The listing builds one solid part. Answer for the finished solid, in the listing's coordinates (mm). Round coordinates to 2 decimals unless told otherwise and drop trailing zeros. Write each loop counter-clockwise with the first axis right and the second up, starting at its lowest first coordinate (ties: lowest second). Pieces come first, ordered by that corner, then holes. Notation, with made-up numbers: (81, 72.5) - (88, 72.5) arc R31 ccw to (88, 101.5) - close; hole circle Ø1 at (30, 70.25). An arc over 180 degrees is marked (long way). Return JSON: item names as keys, results as strings. Group by question number.
(1) Each of these flat-tipped pins is pushed along its axis until it touches: pin 1 (1.5 mm diameter, centred on x = -7.5, y = 1.5, fed in from -Z); pin 2 (1 mm diameter, centred on x = 3.5, y = 0.5, fed in from +Z); pin 3 (1 mm diameter, centred on x = 35, y = 1.5, fed in from -Z). Where does it stop, or does it pass through?
(2) Find the intervals of material crossed by line 1 along Z through (x, y) = (-46.75, 0.7); line 2 along Z through (x, y) = (46.75, 2); line 3 along Z through (x, y) = (-18, 1.4), in increasing order. Write a range as [from, to].
(3) Section D-D, the plane x = -24 is taken. Write down the section's boundary in (y, z), then the cut area to 3 significant figures.
(4) Section B-B, the plane y = 1.6 is taken. Write down the section's boundary in (x, z), then the cut area to 3 significant figures.
(5) Section A-A, the plane x = 46.75 is taken. Write down the section's boundary in (y, z), then the cut area to 3 significant figures.
(6) Section C-C, the plane z = 5.25 is taken. Write down the section's boundary in (x, y).
```python
from build123d import *

# Parameters (mm, degrees)
BOSS_EXTRUDE1_DEPTH = 2.5
CUT_EXTRUDE1_REACH  = 4.5
SKETCH2_R           = 0.5
SKETCH2_R_2         = 1.5


with BuildPart() as part:
    # Sketch1 → Boss-Extrude1 (new body)
    with BuildSketch(Plane(origin=(0, 0, 0), x_dir=(1, 0, 0), z_dir=(0, 1, 0))):
        with BuildLine():
            Line((39.640142036, 3.25), (-43.719713181, 2))
            ThreePointArc((-43.719713181, 2), (-44.367984766, 2.097743563), (-44.949820159, 2.399865109))
            ThreePointArc((-44.949820159, 2.399865109), (-49.75, 0), (-44.949820159, -2.399865109))
            ThreePointArc((-44.949820159, -2.399865109), (-44.367984766, -2.097743563), (-43.719713181, -2))
            Line((-43.719713181, -2), (39.640142036, -3.25))
            ThreePointArc((39.640142036, -3.25), (40.856423208, -3.52767477), (41.854584123, -4.276085054))
            ThreePointArc((41.854584123, -4.276085054), (53.25, 0), (41.854584123, 4.276085054))
            ThreePointArc((41.854584123, 4.276085054), (40.856423208, 3.52767477), (39.640142036, 3.25))
        make_face()
    extrude(amount=BOSS_EXTRUDE1_DEPTH)

    # Sketch2 → Cut-Extrude1 (cut, up to next)
    with BuildSketch(Plane(origin=(0, 2.5, 0), x_dir=(1, 0, 0), z_dir=(0, 1, 0)), mode=Mode.PRIVATE) as cut_extrude1_sk1:
        with Locations((-46.75, 0)):
            Circle(SKETCH2_R)
    cut_extrude1_tool1 = extrude(cut_extrude1_sk1.sketch, amount=-CUT_EXTRUDE1_REACH, mode=Mode.PRIVATE) & part.part
    add(cut_extrude1_tool1.solids().sort_by_distance((-46.75, 2.5, 0))[0], mode=Mode.SUBTRACT)
    # Sketch2 → Cut-Extrude1 (cut, up to next)
    with BuildSketch(Plane(origin=(0, 2.5, 0), x_dir=(1, 0, 0), z_dir=(0, 1, 0)), mode=Mode.PRIVATE) as cut_extrude1_sk2:
        with Locations((46.75, 0)):
            Circle(SKETCH2_R_2)
    cut_extrude1_tool2 = extrude(cut_extrude1_sk2.sketch, amount=-CUT_EXTRUDE1_REACH, mode=Mode.PRIVATE) & part.part
    add(cut_extrude1_tool2.solids().sort_by_distance((46.75, 2.5, 0))[0], mode=Mode.SUBTRACT)


solid = part.part
```
Working result:
{
 "1": {"pin 1": "stops at z = -2.55", "pin 2": "stops at z = 2.72", "pin 3": "stops at z = -3.19"},
 "2": {"line 1": "z = [-3, -0.5], [0.5, 3]", "line 2": "z = [-6.5, -1.5], [1.5, 6.5]", "line 3": "z = [-2.39, 2.39]"},
 "3": {"outline": "(0, -2.3) - (2.5, -2.3) - (2.5, 2.3) - (0, 2.3) - close", "area": "11.5 mm^2"},
 "4": {"outline": "(-44.95, -2.4) arc R2 cw to (-43.72, -2) - (39.64, -3.25) arc R3 cw to (41.85, -4.28) arc R6.5 ccw (long way) to (41.85, 4.28) arc R3 cw to (39.64, 3.25) - (-43.72, 2) arc R2 cw to (-44.95, 2.4) arc R3 ccw (long way) to start; hole circle Ø1 at (-46.75, 0); hole circle Ø3 at (46.75, 0)", "area": "598 mm^2"},
 "5": {"outline": "(0, -6.5) - (2.5, -6.5) - (2.5, -1.5) - (0, -1.5) - close; (0, 1.5) - (2.5, 1.5) - (2.5, 6.5) - (0, 6.5) - close", "area": "25.0 mm^2"},
 "6": {"outline": "(42.92, 0) - (50.58, 0) - (50.58, 2.5) - (42.92, 2.5) - close"}
}
